CAD build for the part. Positions are in the model's coordinates, mm. A direction names the side the tool comes from. Coordinates: 2 decimals unless noted, no trailing zeros. Order: outer loops, then holes, each group sorted by start corner. A loop starts at its lowest first (then second) coordinate and runs counter-clockwise, first axis right, second up. Notation, with made-up numbers: M -19,47 L -4,47 A21 ccw -4,81 Z; hole C 55,52.25 d9. An arc over 180 degrees is marked long. One line per item, written item: value.
from build123d import *

# Parameters (mm, degrees)
SKETCH_1_W          = 86
SKETCH_1_H          = 55.5
EXTRUDE_1_DEPTH     = 8
SKETCH_2_R          = 2.5
CUT_EXTRUDE_1_DEPTH = 25
SKETCH_3_W          = 50
SKETCH_3_H          = 55.5
CUT_EXTRUDE_2_DEPTH = 5
SKETCH_4_R          = 2
CUT_EXTRUDE_3_DEPTH = 103.665719693


with BuildPart() as part:
    # 草图1 → 拉伸1 (new body)
    with BuildSketch(Plane.XY):
        with Locations((43, 27.75)):
            Rectangle(SKETCH_1_W, SKETCH_1_H)
    extrude(amount=EXTRUDE_1_DEPTH)

    # 草图2 → 切除-拉伸1 (cut)
    with BuildSketch(Plane(origin=(0, 55.5, 0), x_dir=(-1, 0, 0), z_dir=(0, 1, 0))):
        with Locations(Location((-78, 4, 0), (0, 0, 90))):
            Circle(SKETCH_2_R)
        with Locations(Location((-8, 4, 0), (0, 0, 90))):
            Circle(SKETCH_2_R)
    extrude(amount=-CUT_EXTRUDE_1_DEPTH, mode=Mode.SUBTRACT)

    # 草图3 → 切除-拉伸2 (cut)
    with BuildSketch(Plane(origin=(0, 0, 0), x_dir=(-1, 0, 0), z_dir=(0, 0, -1))):
        with Locations((-43, 27.75)):
            Rectangle(SKETCH_3_W, SKETCH_3_H)
    extrude(amount=-CUT_EXTRUDE_2_DEPTH, mode=Mode.SUBTRACT)

    # 草图4 → 切除-拉伸3 (cut, through all)
    with BuildSketch(Plane(origin=(0, 0, 0), x_dir=(-1, 0, 0), z_dir=(0, 0, -1))):
        with Locations((-72, 40.5)):
            Circle(SKETCH_4_R)
        with Locations((-78, 10)):
            Circle(SKETCH_4_R)
        with Locations((-14, 40.5)):
            Circle(SKETCH_4_R)
        with Locations((-8, 10)):
            Circle(SKETCH_4_R)
    extrude(amount=-CUT_EXTRUDE_3_DEPTH, mode=Mode.SUBTRACT)


solid = part.part
Q1. Slice it at A-A (z = 4). List the corners of the cut face in (x, y).
Recorded:
outline: M 0,0 L 18,0 L 18,55.5 L 10.5,55.5 L 10.5,30.5 L 5.5,30.5 L 5.5,55.5 L 0,55.5 Z; M 68,0 L 86,0 L 86,55.5 L 80.5,55.5 L 80.5,30.5 L 75.5,30.5 L 75.5,55.5 L 68,55.5 Z; hole C 8,10 d4; hole C 14,40.5 d4; hole C 72,40.5 d4; hole C 78,10 d4
Q2. Slice it at B-B (y = 40.5). List the corners of the cut face in (x, z).
Recorded:
outline: M 0,0 L 12,0 L 12,8 L 0,8 Z; M 16,0 L 18,0 L 18,5 L 68,5 L 68,0 L 70,0 L 70,8 L 16,8 Z; M 74,0 L 86,0 L 86,8 L 74,8 Z; hole C 8,4 d5; hole C 78,4 d5
Q3. Slice it at C-C (x = 14). List the corners of the cut face in (y, z), plus the area to 3 significant figures.
Recorded:
outline: M 0,0 L 38.5,0 L 38.5,8 L 0,8 Z; M 42.5,0 L 55.5,0 L 55.5,8 L 42.5,8 Z
area: 412 mm^2
Q4. Which spindle directions (+Z, -Z, +X, -X, +Y, -Y) get a long thin tool onto all of the face, cutting with end or side? Do faces 1 (the face through (43, 28, 5)), 2 (the face through (78, 30.5, 4)), 3 (the face through (77, 28, 0)). Say none if no direction does.
Recorded:
face 1: -Z, +Y, -Y
face 2: +Y
face 3: -Z, +X, -X, +Y, -Y
Q5. Slice it at D-D (y = 10). List the corners of the cut face in (x, z), plus the area to 3 significant figures.
Recorded:
outline: M 0,0 L 6,0 L 6,8 L 0,8 Z; M 10,0 L 18,0 L 18,5 L 68,5 L 68,0 L 76,0 L 76,8 L 10,8 Z; M 80,0 L 86,0 L 86,8 L 80,8 Z
area: 374 mm^2
Q6. Drill centre lines: line 1 along X through (y, z) = (31, 1.25); line 2 along X through (y, z) = (42, 6); line 3 along X through (y, z) = (41.5, 4.5). Where is each one in solid material? Low to high.
Recorded:
line 1: x = 0 to 18, 68 to 86
line 2: x = 0 to 6.5, 9.5 to 12.68, 15.32 to 70.68, 73.32 to 76.5, 79.5 to 86
line 3: x = 0 to 5.55, 10.45 to 12.27, 15.73 to 18, 68 to 70.27, 73.73 to 75.55, 80.45 to 86
Q7. Mould opens along X. For faces 4 (the face through (0, 27, 4)), 5 (the face through (42, 55.5, 6)), 6 (the face through (68, 27, 2)), 7 (the face through (86, 27, 4)) say: released by +X, released by -X, zero draft, split by the parting line, or undercut.
Recorded:
face 4: released by -X
face 5: zero draft
face 6: undercut
face 7: released by +X
Q8. Pin check, flat tips, straight feed: pin 1 Ø3 at (x, y) = (14, 40.5) entering from -Z; pin 2 Ø3 at (x, z) = (8, 4) entering from +Y; pin 3 Ø2 at (x, y) = (43, 45.5) entering from -Z. Stop position of each tip, or through.
Recorded:
pin 1: passes through
pin 2: stops at y = 30.5
pin 3: stops at z = 5
